Drawing for the job (mm, zero at the part's lowest x, y, z). Give positions to 0.01 mm unless a question says otherwise; leave off trailing zeros. Loops run counter-clockwise (first coordinate to the right, second up) from the corner with the lowest first, then second, coordinate; pieces in that order, holes last. Notation, with made-up numbers: (78.25, 57.5) -> (106.25, 57.5) arc R22 ccw to (106.25, 68.5) -> close; hole circle Ø11 at (53.25, 58). An arc over 180 degrees is marked (long way). Answer in a Markdown table with one row per item. Add a question column.
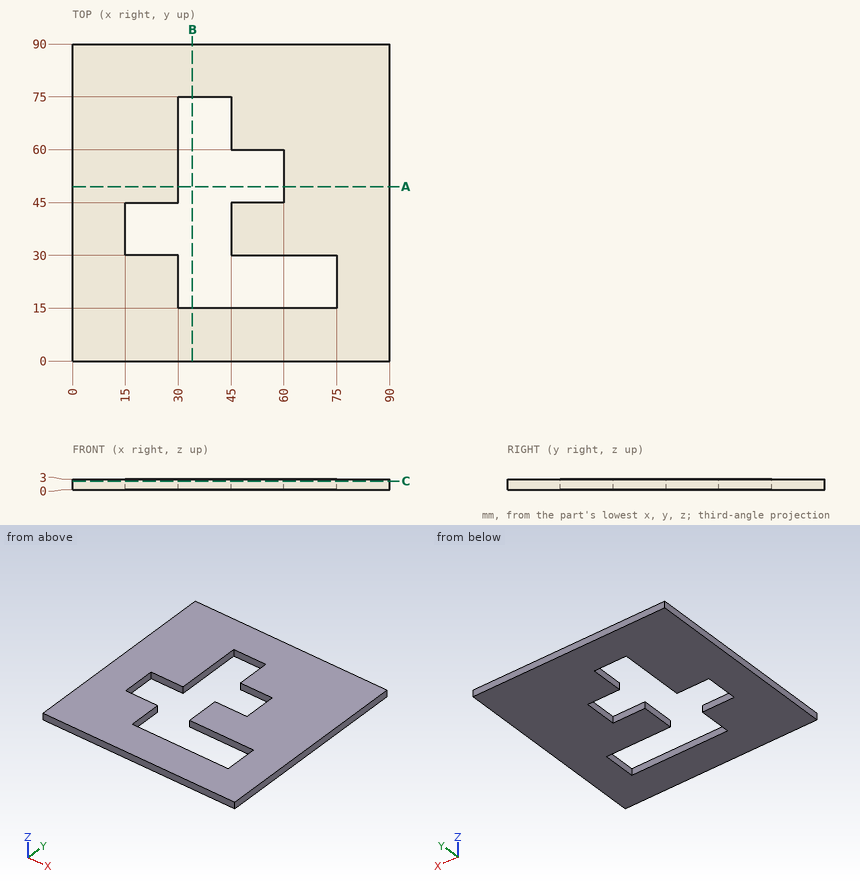
(1) Saw through at A-A, the plane y = 49.5. List the corners of the cut face in (x, z), then the cut area to 3 significant figures.
(2) Saw through at C-C, the plane z = 2.4. List the corners of the cut face in (x, y), then the cut area to 3 significant figures.
(3) Wall check: line 1 along Y through (x, z) = (51, 2.15); line 2 along Y through (x, z) = (72, 2.5); line 3 along X through (y, z) = (74.5, 1.4). Give the ranges that are in metal, low to high. Write a range as from..to.
(4) Saw through at B-B, the plane x = 34. List the corners of the cut face in (y, z), then the cut area to 3 significant figures.
Worked answers:
| question | item | result |
|---|---|---|
| 1 | outline | (0, 0) -> (30, 0) -> (30, 3) -> (0, 3) -> close; (60, 0) -> (90, 0) -> (90, 3) -> (60, 3) -> close |
| 1 | area | 180 mm^2 |
| 2 | outline | (0, 0) -> (90, 0) -> (90, 90) -> (0, 90) -> close; hole (15, 30) -> (30, 30) -> (30, 15) -> (75, 15) -> (75, 30) -> (45, 30) -> (45, 45) -> (60, 45) -> (60, 60) -> (45, 60) -> (45, 75) -> (30, 75) -> (30, 45) -> (15, 45) -> close |
| 2 | area | 6,300 mm^2 |
| 3 | line 1 | 0..15, 30..45, 60..90 |
| 3 | line 2 | 0..15, 30..90 |
| 3 | line 3 | 0..30, 45..90 |
| 4 | outline | (0, 0) -> (15, 0) -> (15, 3) -> (0, 3) -> close; (75, 0) -> (90, 0) -> (90, 3) -> (75, 3) -> close |
| 4 | area | 90.0 mm^2 |
